Autodesk Inventor part; units mm, degrees
ref_plane "YZ Plane" through (0, 0, 0) normal (1, 0, 0) x (0, 1, 0)
ref_plane "XZ Plane" through (0, 0, 0) normal (0, 1, 0) x (-1, 0, 0)
ref_plane "XY Plane" through (0, 0, 0) normal (0, 0, 1) x (1, 0, 0)
sketch "Sketch1" plane through (0, 0, 0) normal (0, 0, 1) x (1, 0, 0)
  line L0 (-19.225, -30) -> (-22.225, -30) construction
  line L1 (-22.225, -30) -> (-22.225, -20) construction
  line L2 (-22.225, -20) -> (-19.225, -20) construction
  line L3 (-19.225, -20) -> (-19.225, -30) construction
  line L4 (-22, 36.7378) -> (-19.225, 21)
  line L5 (-22.5, 0) -> (-22.5, 23.7378)
  line L6 (-22.5, 23.7378) -> (-21.5, 23.7378)
  line L7 (-21.5, 23.7378) -> (-21.5, 25.7378)
  line L8 (-21.5, 25.7378) -> (-22.5, 25.7378)
  line L9 (-22.5, 25.7378) -> (-22.5, 36.7378)
  line L10 (-22, 36.7378) -> (-22.5, 36.7378)
  line L11 (0, -43.3476) -> (0, 50.0854)
  line L12 (-19.225, -20) -> (-20.225, -20) construction
  line L13 (-20.225, -20) -> (-20.225, 0) construction
  line L14 (-20.225, 0) -> (-19.225, 0) construction
  line L15 (-19.225, 0) -> (-19.225, -20) construction
  line L16 (-22.5, 0) -> (-20.225, 0)
  line L17 (-20.225, 0) -> (-20.225, 21)
  line L18 (-20.225, 21) -> (-19.225, 21)
  point P0 (0, 0)
  dimension "d0" = 10
  dimension "d1" = 22.225
  dimension "d3" = 3
  dimension "d5" = 11
  dimension "d6" = 2
  dimension "d7" = 22.5
  dimension "d10" = 21
  dimension "d12" = 1
  dimension "d16" = 20
  dimension "d17" = 1
  dimension "d18" = 0.5
  dimension "d19" = 10
revolve "Revolution1" add sketch "Sketch1" angle 360 about axis through (0, -10, 0) along (0, 1, 0)
properties part number "CapCone" material "Brass, Soft Yellow, Welded"
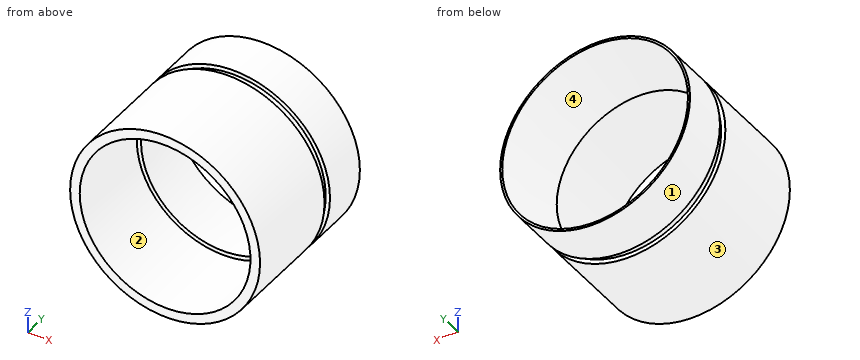
Input: part model. Units: mm. Frame: model coordinates. Face numbers are marked on the shaded views. A direction names the side the tool comes from. Give positions to 0.01 mm unless a question says otherwise; leave off trailing zeros. Order: outer loops, then holes, each group sorted by start corner. A loop starts at its lowest first (then second) coordinate and runs counter-clockwise, first axis right, second up. Notation, with made-up numbers: M -35,-38.5 L 8,-38.5 A22 ccw 8,-30.5 Z; hole C -30.5,25 d4. An arc over 180 degrees is marked long. Return JSON: item names as keys, results as strings.
1) Contact query for flat-ended pins moving along their axis: pin 1 (2 mm diameter, centred on x = 3, y = 4, fed in from +Z); pin 2 (12 mm diameter, centred on x = 17.5, y = 14, fed in from -Z); pin 3 (1 mm diameter, centred on x = -9.5, y = 14, fed in from +Z); pin 4 (22.5 mm diameter, centred on x = -4, z = 9.5, fed in from -Y). Output: stop coordinate, or through.
Taken from the geometry:
{"pin 1": "stops at z = 22.41", "pin 2": "stops at z = -19.34", "pin 3": "stops at z = 20.62", "pin 4": "stops at y = 0"}
2) Section query C-C on y = 23. Output: boundary loops of the cut face in (x, z), and give its area (3 significant figures).
Taken from the geometry:
{"outline": "C 0,0 d45; hole C 0,0 d39.16", "area": "386 mm2"}
3) Mould query, pull axis Z, two halves, no side actions, for the marked faces 3 and 4. Classes: released by +Z, released by -Z, zero draft, split by the parting line, or undercut.
Taken from the geometry:
{"face 3": "split by the parting line", "face 4": "undercut"}
4) Line query: L1, parallel to Z at x = 0, y = 12 (3 decimals); L2, parallel to Y at x = 12, z = 18.5; L3, parallel to Z at x = -7, y = 28. Output: solid intervals per line, ascending. Write a range as [from, to].
Taken from the geometry:
{"L1": "z = [-22.5, -20.225], [20.225, 22.5]", "L2": "y = [0, 23.74], [25.74, 36.74]", "L3": "z = [-21.38, -19.22], [19.22, 21.38]"}
5) Section query A-A on x = 0. Output: boundary loops of the cut face in (y, z) (3 decimals), and give its area (3 significant figures).
Taken from the geometry:
{"outline": "M 0,-22.5 L 23.738,-22.5 L 23.738,-21.5 L 25.738,-21.5 L 25.738,-22.5 L 36.738,-22.5 L 36.738,-22 L 21,-19.225 L 21,-20.225 L 0,-20.225 Z; M 0,20.225 L 21,20.225 L 21,19.225 L 36.738,22 L 36.738,22.5 L 25.738,22.5 L 25.738,21.5 L 23.738,21.5 L 23.738,22.5 L 0,22.5 Z", "area": "151 mm2"}
6) Section query B-B on z = 0. Output: boundary loops of the cut face in (x, y) (3 decimals), and give its area (3 significant figures).
Taken from the geometry:
{"outline": "M -22.5,0 L -20.225,0 L -20.225,21 L -19.225,21 L -22,36.738 L -22.5,36.738 L -22.5,25.738 L -21.5,25.738 L -21.5,23.738 L -22.5,23.738 Z; M 19.225,21 L 20.225,21 L 20.225,0 L 22.5,0 L 22.5,23.738 L 21.5,23.738 L 21.5,25.738 L 22.5,25.738 L 22.5,36.738 L 22,36.738 Z", "area": "151 mm2"}
7) Access query for the marked faces 1 and 2. Directions: +Z, -Z, +X, -X, +Y, -Y. A direction counts if a zero-diameter tool reaches every point of the face in a straight line with its end or side. Return the directions, or none.
Taken from the geometry:
{"face 1": "+Y, -Y", "face 2": "-Y"}
